The listing builds one solid part. Answer for the finished solid, in the listing's coordinates (mm). Give positions to 0.01 mm unless a question says otherwise; leave off trailing zeros. Order: outer loops, then holes, each group sorted by start corner. A loop starts at its lowest first (then second) coordinate and runs counter-clockwise, first axis right, second up. Notation, with made-up numbers: (75.5, 87.5) - (93.5, 87.5) arc R31 ccw to (93.5, 126.5) - close; hole circle Ø5 at (-37, 1). An arc over 180 degrees is marked (long way). Answer as CSV lines item,"result". Start each with the question number.
1. A flat-ended cylindrical pin translates along its axis: pin 1 (1.1 mm diameter, centred on x = 48.9, z = 5.4, fed in from +Y). Find the tip coordinate at first contact, or state that the pin passes through.
2. Section B-B on z = 0 is taken. Give the vertices of the cut face in (x, y), and give its area (3 significant figures).
3. Consider line 1 along Z through (x, y) = (-11.43, -0.15); line 2 along X through (y, z) = (-0.35, 0); line 3 along X through (y, z) = (-0.6, -5). Determine where each line is inside the solid, lowest interval first. Write a range as [from, to].
4. Section A-A on x = -11.43 is taken. Give the vertices of the cut face in (y, z).
Autodesk Inventor part; units mm, degrees
ref_plane "YZ Plane" through (0, 0, 0) normal (1, 0, 0) x (0, 1, 0)
ref_plane "XZ Plane" through (0, 0, 0) normal (0, 1, 0) x (-1, 0, 0)
ref_plane "XY Plane" through (0, 0, 0) normal (0, 0, 1) x (1, 0, 0)
sketch "Sketch1" plane through (0, 0, 0) normal (0, 1, 0) x (-1, 0, 0)
  line L0 (0, -13.3) -> (0, 13.3)
  line L1 (-72.898, 0) -> (72.898, 0)
  line L2 (-52.07, -9.5) -> (52.07, -9.5)
  line L3 (52.07, -9.5) -> (52.07, 9.5)
  line L4 (52.07, 9.5) -> (-52.07, 9.5)
  line L5 (-52.07, 9.5) -> (-52.07, -9.5)
  line L6 (-52.07, -9.5) -> (52.07, 9.5) construction
  line L7 (52.07, -9.5) -> (-52.07, 9.5) construction
  point P0 (0, 0)
  point P1 (11.43, 0)
  point P2 (-48.895, 5.3975)
  point P3 (-48.895, -5.3975)
  dimension "d0" = 19
  dimension "d1" = 104.14
  dimension "d2" = 40.64
  dimension "d13" = 10.795
  dimension "d14" = 5.3975
  dimension "d15" = 3.175
extrude "Extrusion1" add sketch "Sketch1" against normal blind 0.762
hole "Hole1" at (-11.43, 0, 0) direction (0, -1, 0) diameter 1.7145 end through all
fillet "Fillet1" radius 1.905 4 edges at (-52.07, -0.381, 9.5) (-52.07, -0.381, -9.5) (52.07, -0.381, 9.5) (52.07, -0.381, -9.5)
hole "Hole2" at (48.895, 0, 5.3975) at (48.895, 0, -5.3975) direction (0, -1, 0) diameter 1.778 end through all countersink diameter 3.0226 countersink angle 82
sketch "Sketch3" plane through (0, 0, 0) normal (0, 1, 0) x (-1, 0, 0)
  line L0 (0, -2.6111) -> (0, 15.6667)
  line L1 (-44.958, 0) -> (7.493, 0)
  circle A0 centre (-35.052, 10.6426) radius 2.413
  point P0 (0, 0)
  dimension "d26" = 4.826
  dimension "d27" = 35.052
  dimension "d28" = 10.6426
extrude "Extrusion2" cut sketch "Sketch3" against normal through all
mirror "Mirror2" about plane through (0, 0, 0) normal (0, 0, 1) of "Extrusion2"
fillet "Fillet2" radius 0.635 4 edges at (32.9267, -0.381, -9.5) (37.1773, -0.381, -9.5) (37.1773, -0.381, 9.5) (32.9267, -0.381, 9.5)
properties part number "J010356" material "POLYCARBONATE, CLEAR"
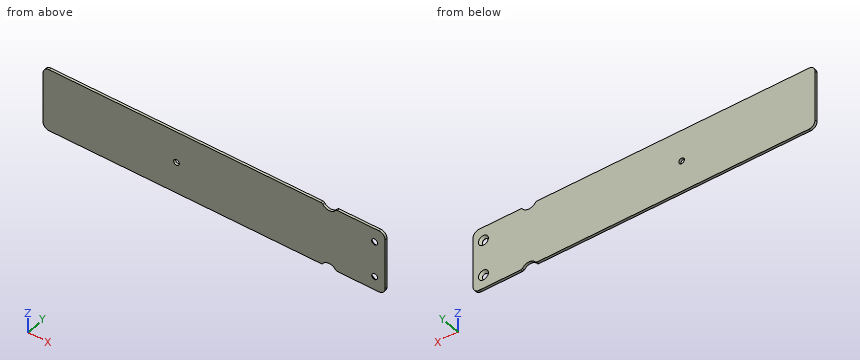
Checks:
1,pin 1,"passes through"
2,outline,"(-52.07, -0.76) - (-12.29, -0.76) - (-12.29, 0) - (-52.07, 0) - close; (-10.57, -0.76) - (52.07, -0.76) - (52.07, 0) - (-10.57, 0) - close"
2,area,"78.0 mm²"
3,line 1,"z = [-9.5, -0.86], [0.86, 9.5]"
3,line 2,"x = [-52.07, -12.29], [-10.57, 52.07]"
3,line 3,"x = [-52.07, 47.99], [49.8, 52.07]"
4,outline,"(-0.76, -9.5) - (0, -9.5) - (0, -0.86) - (-0.76, -0.86) - close; (-0.76, 0.86) - (0, 0.86) - (0, 9.5) - (-0.76, 9.5) - close"
